Work out the finished part from the listing and answer in its coordinate system (mm). A direction names the side the tool comes from. Give positions to 0.01 mm unless a question says otherwise; leave off trailing zeros. Loops run counter-clockwise (first coordinate to the right, second up) from the corner with the lowest first, then second, coordinate; pieces in that order, holes last. Notation, with made-up numbers: (7, -36.5) - (12, -36.5) arc R30 ccw to (12, -7.5) - close; hole circle Ø9 at (16, 31.25). An arc over 180 degrees is marked (long way). One line per item, written item: value.
from build123d import *

# Parameters (mm, degrees)
BOSS_EXTRUDE1_DEPTH      = 12.7
BOSS_EXTRUDE2_DEPTH      = 57.15
BOSS_EXTRUDE2_DEPTH_BACK = 57.15
SKETCH8_R                = 9.525
CUT_EXTRUDE2_DEPTH       = 170.081792337
SKETCH9_W                = 139.7
SKETCH9_H                = 63.5
CUT_EXTRUDE3_DEPTH       = 196.926057481
FILLET1_R                = 6.35
SKETCH10_R               = 6.35
CUT_EXTRUDE4_DEPTH       = 164.751221369


with BuildPart() as part:
    # Sketch1 → Boss-Extrude1 (new body)
    with BuildSketch(Plane(origin=(0, 0, 0), x_dir=(1, 0, 0), z_dir=(0, 1, 0))):
        with BuildLine():
            Line((101.6, 38.1), (-101.6, 38.1))
            ThreePointArc((-101.6, 38.1), (-74.659231637, 26.940768363), (-63.5, 0))
            ThreePointArc((-63.5, 0), (-74.659231637, -26.940768363), (-101.6, -38.1))
            Line((-101.6, -38.1), (101.6, -38.1))
            ThreePointArc((101.6, -38.1), (63.5, 0), (101.6, 38.1))
        make_face()
        with BuildLine():
            ThreePointArc((-63.5, 0), (-74.659231637, 26.940768363), (-101.6, 38.1))
            Line((-101.6, 38.1), (-101.6, -38.1))
            ThreePointArc((-101.6, -38.1), (-74.659231637, -26.940768363), (-63.5, 0))
        make_face()
        with BuildLine():
            Line((-101.6, -38.1), (-101.6, 38.1))
            ThreePointArc((-101.6, 38.1), (-139.7, 0), (-101.6, -38.1))
        make_face()
        with BuildLine():
            ThreePointArc((139.7, 0), (128.540768363, 26.940768363), (101.6, 38.1))
            Line((101.6, 38.1), (101.6, -38.1))
            ThreePointArc((101.6, -38.1), (128.540768363, -26.940768363), (139.7, 0))
        make_face()
        with BuildLine():
            Line((101.6, -38.1), (101.6, 38.1))
            ThreePointArc((101.6, 38.1), (63.5, 0), (101.6, -38.1))
        make_face()
    extrude(amount=BOSS_EXTRUDE1_DEPTH)

    # Sketch2 → Boss-Extrude2 (add, two sides: drawn at the far end of the back side and taken through both)
    with BuildSketch(Plane.XY.offset(-BOSS_EXTRUDE2_DEPTH_BACK)):
        Polygon((69.85, 0), (69.85, 63.5), (-69.85, 63.5), (-69.85, 0), (-82.55, 0), (-82.55, 76.2), (82.55, 76.2), (82.55, 0), align=None)
    extrude(amount=BOSS_EXTRUDE2_DEPTH + BOSS_EXTRUDE2_DEPTH_BACK)

    # Sketch8 → Cut-Extrude2 (cut, through all)
    with BuildSketch(Plane(origin=(0, 0, 0), x_dir=(1, 0, 0), z_dir=(0, 1, 0))):
        with Locations(Location((0, 0, 0), (0, 0, 90))):
            Circle(SKETCH8_R)
    extrude(amount=CUT_EXTRUDE2_DEPTH, mode=Mode.SUBTRACT)

    # Sketch9 → Cut-Extrude3 (cut, through all)
    with BuildSketch(Plane.XY.offset(57.15)):
        with Locations((0, 31.75)):
            Rectangle(SKETCH9_W, SKETCH9_H)
    extrude(amount=-CUT_EXTRUDE3_DEPTH, mode=Mode.SUBTRACT)

    # Fillet1
    fillet1_edges = [part.edges().sort_by_distance(p)[0] for p in [
        (-69.85, 63.5, 0),
        (82.55, 76.2, 0),
        (69.85, 63.5, 0),
        (-82.55, 76.2, 0),
    ]]
    fillet(fillet1_edges, radius=FILLET1_R)

    # Sketch10 → Cut-Extrude4 (cut, through all)
    with BuildSketch(Plane(origin=(0, 12.7, 0), x_dir=(1, 0, 0), z_dir=(0, 1, 0))):
        with Locations(Location((101.6, 0, 0), (0, 0, 270))):
            Circle(SKETCH10_R)
        with Locations(Location((-101.6, 0, 0), (0, 0, 270))):
            Circle(SKETCH10_R)
    extrude(amount=-CUT_EXTRUDE4_DEPTH, mode=Mode.SUBTRACT)


solid = part.part
1. Flat-ended cylindrical pins translate along their axes: pin 1 Ø12 at (y, z) = (13.5, -3.5) entering from -X; pin 2 Ø4 at (x, y) = (-94.5, 8) entering from -Z; pin 3 Ø17 at (x, z) = (123.5, 8) entering from +Y. Find the tip coordinate at first contact, or state that the pin passes through.
Output:
pin 1: stops at x = -139.7
pin 2: stops at z = -38.1
pin 3: stops at y = 12.7
2. Section C-C (z = 42) is taken. Write down the section's boundary in (x, y), and give its area (3 significant figures).
Output:
outline: (-82.55, 0) - (-69.85, 0) - (-69.85, 57.15) arc R6.35 cw to (-63.5, 63.5) - (63.5, 63.5) arc R6.35 cw to (69.85, 57.15) - (69.85, 0) - (82.55, 0) - (82.55, 69.85) arc R6.35 ccw to (76.2, 76.2) - (-76.2, 76.2) arc R6.35 ccw to (-82.55, 69.85) - close
area: 3,710 mm²
3. Section A-A (y = 53.5) is taken. Write down the section's boundary in (x, z), and give its area (3 significant figures).
Output:
outline: (-82.55, -57.15) - (-69.85, -57.15) - (-69.85, 57.15) - (-82.55, 57.15) - close; (69.85, -57.15) - (82.55, -57.15) - (82.55, 57.15) - (69.85, 57.15) - close
area: 2,900 mm²
4. For faces 1 (the flat face through (-92, 6, 38.1)), 2 (the cylindrical face through (-67.94, 61.69, 0.8)), 3 (the flat face through (-92, 6, -38.1)), 4 (the flat face through (111, 12.7, -1)), 5 (the flat face through (92, 6, 38.1)), determine the directions among +Z, -Z, +X, -X, +Y, -Y from which every point of the face is accessible in a straight line to the end or side of a thin tool.
Output:
face 1: +Z, -X, +Y, -Y
face 2: +Z, -Z, -Y
face 3: -Z, -X, +Y, -Y
face 4: +Z, -Z, +X, +Y
face 5: +Z, +X, +Y, -Y
5. Section D-D (z = -3) is taken. Write down the section's boundary in (x, y), and give its area (3 significant figures).
Output:
outline: (-139.58, 0) - (-107.2, 0) - (-107.2, 12.7) - (-139.58, 12.7) - close; (-96, 0) - (-69.85, 0) - (-69.85, 57.15) arc R6.35 cw to (-63.5, 63.5) - (-9.04, 63.5) - (-9.04, 76.2) - (-76.2, 76.2) arc R6.35 ccw to (-82.55, 69.85) - (-82.55, 12.7) - (-96, 12.7) - close; (9.04, 63.5) - (63.5, 63.5) arc R6.35 cw to (69.85, 57.15) - (69.85, 0) - (96, 0) - (96, 12.7) - (82.55, 12.7) - (82.55, 69.85) arc R6.35 ccw to (76.2, 76.2) - (9.04, 76.2) - close; (107.2, 0) - (139.58, 0) - (139.58, 12.7) - (107.2, 12.7) - close
area: 4,640 mm²
6. The mould has two halves that part along X. Classify faces 6 (the cylindrical face through (-139.69, 6.26, -0.84)), 7 (the cylindrical face through (107.9, 6.4, -0.8)), 8 (the cylindrical face through (80.64, 74.39, 0.8)), 9 (the flat face through (-112, 12.7, -1)): released by +X, released by -X, zero draft, split by the parting line, or undercut.
Output:
face 6: released by -X
face 7: undercut
face 8: released by +X
face 9: zero draft
7. Section B-B (x = 0) is taken. Write down the section's boundary in (y, z) (3 decimals), and give its area (3 significant figures).
Output:
outline: (63.5, -57.15) - (76.2, -57.15) - (76.2, -9.525) - (63.5, -9.525) - close; (63.5, 9.525) - (76.2, 9.525) - (76.2, 57.15) - (63.5, 57.15) - close
area: 1,210 mm²
8. Find the intervals of material crossed by line 1 along X through (y, z) = (47.5, 0); line 2 along X through (y, z) = (69, 0) (3 decimals); line 3 along Z through (x, y) = (101, 5), in increasing order.
Output:
line 1: x = -82.55 to -69.85, 69.85 to 82.55
line 2: x = -82.55 to -9.525, 9.525 to 82.55
line 3: z = -38.1 to -6.32, 6.32 to 38.1
